from build123d import *

# Parameters (mm, degrees)
SKETCH_W        = 150
SKETCH_H        = 145
PAD_DEPTH       = 5
SKETCH001_R     = 1.519453
SKETCH001_R_2   = 1.575641
SKETCH001_R_3   = 1.584812
SKETCH001_R_4   = 1.460672
POCKET_DEPTH    = 5
SKETCH003_R     = 3
SKETCH003_R_2   = 1.5
PAD002_DEPTH    = 5
SKETCH004_W     = 5
SKETCH004_H     = 25
SKETCH004_W_2   = 30
SKETCH004_H_2   = 3
PAD003_DEPTH    = 9
SKETCH005_W     = 7
SKETCH005_H     = 5
PAD004_DEPTH    = 27
PAD003_FACE49_W = 3
PAD003_FACE49_H = 30
PAD006_DEPTH    = 17
SKETCH008_W     = 5
SKETCH008_H     = 7
PAD007_DEPTH    = 15
PAD007_FACE50_W = 5
PAD007_FACE50_H = 7
PAD008_DEPTH    = 17
PAD008_FACE55_W = 3
PAD008_FACE55_H = 30
PAD009_DEPTH    = 14
SKETCH009_W     = 8.674523
SKETCH009_H     = 6.940131
PAD010_DEPTH    = 14
PAD010_FACE69_W = 25
PAD010_FACE69_H = 5
PAD011_DEPTH    = 14
SKETCH012_W     = 5
SKETCH012_H     = 7
SKETCH012_R     = 1.75
PAD013_DEPTH    = 58
FILLET001_R     = 5


with BuildPart() as part:
    # Sketch → Pad (new body)
    with BuildSketch(Plane.XY):
        Rectangle(SKETCH_W, SKETCH_H)
    extrude(amount=-PAD_DEPTH)

    # Sketch001 (on Face5 of Pad) → Pocket (cut)
    with BuildSketch(Plane.XY):
        with Locations((54, 63.26)):
            Circle(SKETCH001_R)
        with Locations((69, 63.26)):
            Circle(SKETCH001_R_2)
        with Locations((69, 49.76)):
            Circle(SKETCH001_R_3)
        with Locations((54, 49.76)):
            Circle(SKETCH001_R_4)
        with Locations((54, -49.76)):
            Circle(SKETCH001_R)
        with Locations((69, -49.76)):
            Circle(SKETCH001_R_2)
        with Locations((69, -63.26)):
            Circle(SKETCH001_R_3)
        with Locations((54, -63.26)):
            Circle(SKETCH001_R_4)
    extrude(amount=-POCKET_DEPTH, mode=Mode.SUBTRACT)

    # Sketch003 (on Face4 of Pocket) → Pad002 (join)
    with BuildSketch(Plane.XY):
        with Locations((69.767639, -18.269884)):
            Circle(SKETCH003_R)
        with Locations((69.767639, -18.269884)):
            Circle(SKETCH003_R_2, mode=Mode.SUBTRACT)
        with Locations((32.256084, -18.291882)):
            Circle(SKETCH003_R)
        with Locations((32.256084, -18.291882)):
            Circle(SKETCH003_R_2, mode=Mode.SUBTRACT)
        with Locations((32.284943, -55.757919)):
            Circle(SKETCH003_R)
        with Locations((32.284943, -55.757919)):
            Circle(SKETCH003_R_2, mode=Mode.SUBTRACT)
        with Locations((69.736526, -55.773216)):
            Circle(SKETCH003_R)
        with Locations((69.736526, -55.773216)):
            Circle(SKETCH003_R_2, mode=Mode.SUBTRACT)
        with Locations((-62.054475, -15.516004)):
            Circle(SKETCH003_R)
        with Locations((-62.054475, -15.516004)):
            Circle(SKETCH003_R_2, mode=Mode.SUBTRACT)
        with Locations((-4.044475, -15.613503)):
            Circle(SKETCH003_R)
        with Locations((-4.044475, -15.613503)):
            Circle(SKETCH003_R_2, mode=Mode.SUBTRACT)
        with Locations((-4.044475, -64.673503)):
            Circle(SKETCH003_R)
        with Locations((-4.044475, -64.673503)):
            Circle(SKETCH003_R_2, mode=Mode.SUBTRACT)
        with Locations((-62.064475, -64.556004)):
            Circle(SKETCH003_R)
        with Locations((-62.064475, -64.556004)):
            Circle(SKETCH003_R_2, mode=Mode.SUBTRACT)
    extrude(amount=PAD002_DEPTH)

    # Sketch004 (on Face4 of Pad002) → Pad003 (join)
    with BuildSketch(Plane.XY):
        with Locations((68.561538, 20.263053)):
            Rectangle(SKETCH004_W, SKETCH004_H)
        with Locations((-71.331904, 45.140981)):
            Rectangle(SKETCH004_W, SKETCH004_H)
        with Locations((-3.448665, 69.481535)):
            Rectangle(SKETCH004_W_2, SKETCH004_H_2)
        with Locations((-3.448665, -7.480191)):
            Rectangle(SKETCH004_W_2, SKETCH004_H_2)
    extrude(amount=PAD003_DEPTH)

    # Sketch005 (on Face4 of Pad003) → Pad004 (join)
    with BuildSketch(Plane.XY):
        with Locations((-40.03, -8.180035)):
            Rectangle(SKETCH005_W, SKETCH005_H)
        with Locations((30.99, -8.180035)):
            Rectangle(SKETCH005_W, SKETCH005_H)
    extrude(amount=PAD004_DEPTH)

    # Pad003 Face49 → Pad006 (add)
    with BuildSketch(Plane(origin=(-3.448665, 69.481535, 9), x_dir=(0, 1, 0), z_dir=(0, 0, 1))):
        Rectangle(PAD003_FACE49_W, PAD003_FACE49_H)
    extrude(amount=PAD006_DEPTH)

    # Sketch008 (on Face60 of Pad006) → Pad007 (join)
    with BuildSketch(Plane.XZ.offset(-67.981535)):
        with Locations((-15.105862, 18.267392)):
            Rectangle(SKETCH008_W, SKETCH008_H)
    extrude(amount=PAD007_DEPTH)

    # Pad007 Face50 → Pad008 (add)
    with BuildSketch(Plane(origin=(-40.03, -8.180035, 27), x_dir=(0, 1, 0), z_dir=(0, 0, 1))):
        Rectangle(PAD007_FACE50_W, PAD007_FACE50_H)
    extrude(amount=PAD008_DEPTH)

    # Pad008 Face55 → Pad009 (add)
    with BuildSketch(Plane(origin=(-3.448665, -7.480191, 9), x_dir=(0, 1, 0), z_dir=(0, 0, 1))):
        Rectangle(PAD008_FACE55_W, PAD008_FACE55_H)
    extrude(amount=PAD009_DEPTH)

    # Sketch009 (on Face58 of Pad009) → Pad010 (join)
    with BuildSketch(Plane(origin=(0, -5.980191, 0), x_dir=(-1, 0, 0), z_dir=(0, 1, 0))):
        with Locations((-6.437226, 17.328186)):
            Rectangle(SKETCH009_W, SKETCH009_H)
    extrude(amount=PAD010_DEPTH)

    # Pad010 Face69 → Pad011 (add)
    with BuildSketch(Plane(origin=(68.561538, 20.263053, 9), x_dir=(0, 1, 0), z_dir=(0, 0, 1))):
        Rectangle(PAD010_FACE69_W, PAD010_FACE69_H)
    extrude(amount=PAD011_DEPTH)

    # Sketch012 (on Face4 of Pad011) → Pad013 (join)
    with BuildSketch(Plane.XY):
        with Locations((-70.126444, -9.436971)):
            Rectangle(SKETCH012_W, SKETCH012_H)
        with Locations((-70.126444, -9.436971)):
            Circle(SKETCH012_R, mode=Mode.SUBTRACT)
        with Locations((67.407579, -9.436971)):
            Rectangle(SKETCH012_W, SKETCH012_H)
        with Locations((67.407579, -9.436971)):
            Circle(SKETCH012_R, mode=Mode.SUBTRACT)
    extrude(amount=PAD013_DEPTH)

    # Fillet001
    fillet001_edges = [part.edges().sort_by_distance(p)[0] for p in [
        (-75, 72.5, -2.5),
        (-75, -72.5, -2.5),
    ]]
    fillet(fillet001_edges, radius=FILLET001_R)


with BuildPart() as part_1:
    # Body001 placement: moved
    add(part.part.moved(Location((11, 0, 0))))


solid = part_1.part
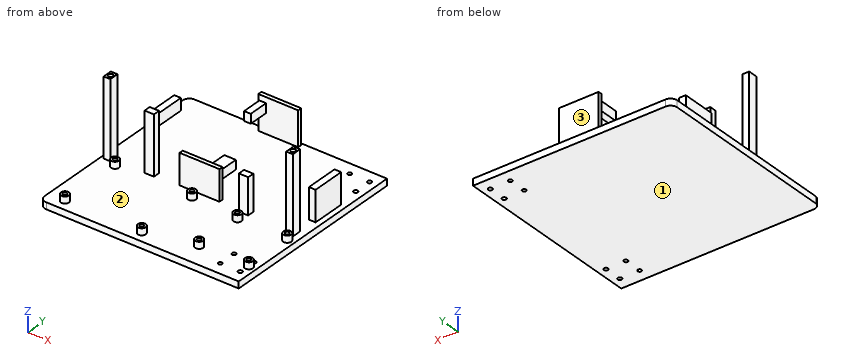
Build history of the part. All positions in model axes, mm. Face numbers are marked on the shaded views. Round coordinates to 2 decimals unless told otherwise and drop trailing zeros. Write each loop counter-clockwise with the first axis right and the second up, starting at its lowest first coordinate (ties: lowest second). Pieces come first, ordered by that corner, then holes. Notation, with made-up numbers: M 26.25,-32 L 61.25,-32 A12 cw 61.25,-25 Z; hole C 42,50.5 d3. An arc over 180 degrees is marked long. Answer as a JSON object with one key per item and string values. Group by question number.
(1) Cut at A-A (z = 47). Give the cut face in (x, y), and give its area (3 significant figures).
(2) Cut at B-B (z = 35). Give the cut face in (x, y), and give its area (3 significant figures).
(3) Mould opens along Y. For the marked faces 1, 2 and 3 say: pulls with the +Y half, pulls with the -Y half, needs draft (parallel to the pull), parting line crosses it, or undercut.
(4) Flat gauge pins, fed straight in: pin 1 (7 mm diameter, centred on x = 4.5, z = 13.5, fed in from +Y); pin 2 (5.5 mm diameter, centred on y = -9, z = 18, fed in from -X); pin 3 (2.5 mm diameter, centred on x = 6.5, y = -15.5, fed in from +Z); pin 4 (10 mm diameter, centred on y = 44.5, z = 2.5, fed in from +X). Where does each tip first touch, or does it go through?
(5) Cut at D-D (y = -42). Give the cut face in (x, z).
(6) Drill centre lines: L1, parallel to Y at x = 65, z = -2.2; L2, parallel to Y at x = 22.5, z = 4; L3, parallel to Z at x = 23, y = -58. Where is each one in solid material? Low to high.
(7) Cut at C-C (x = -10). Give the cut face in (y, z), and give its area (3 significant figures).
Responses:
{
 "1": {"outline": "M -61.63,-12.94 L -56.63,-12.94 L -56.63,-5.94 L -61.63,-5.94 Z; M 75.91,-12.94 L 80.91,-12.94 L 80.91,-5.94 L 75.91,-5.94 Z; hole C -59.13,-9.44 d3.5; hole C 78.41,-9.44 d3.5", "area": "50.8 mm2"},
 "2": {"outline": "M -61.63,-12.94 L -56.63,-12.94 L -56.63,-5.94 L -61.63,-5.94 Z; M -32.53,-10.68 L -25.53,-10.68 L -25.53,-5.68 L -32.53,-5.68 Z; M 75.91,-12.94 L 80.91,-12.94 L 80.91,-5.94 L 75.91,-5.94 Z; hole C -59.13,-9.44 d3.5; hole C 78.41,-9.44 d3.5", "area": "85.8 mm2"},
 "3": {"face 1": "needs draft", "face 2": "undercut", "face 3": "pulls with the +Y half"},
 "4": {"pin 1": "stops at y = 70.98", "pin 2": "stops at x = -61.63", "pin 3": "stops at z = 5", "pin 4": "stops at x = 86"},
 "5": {"outline": "M -64,-5 L 86,-5 L 86,0 L -64,0 Z"},
 "6": {"L1": "y = -72.5 to -64.72, -61.8 to -51.28, -48.24 to 48.3, 51.22 to 61.74, 64.78 to 72.5", "L2": "y = -8.98 to -5.98, 67.98 to 70.98", "L3": "z = -5 to 0"},
 "7": {"outline": "M -72.5,-5 L 72.5,-5 L 72.5,0 L -72.5,0 Z", "area": "725 mm2"}
}
